Can you work these out from the model? Positions are in its coordinate system, mm. Face numbers are marked on the shaded views. A direction names the side the tool comes from. Give positions to 0.01 mm unless a question says otherwise; leave off trailing zeros. Loops run counter-clockwise (first coordinate to the right, second up) from the corner with the lowest first, then second, coordinate; pieces in that order, holes last. Notation, with made-up numbers: M 18,-20 L 30,-20 A29 ccw 30,17 Z; hole C 85.5,48 d10. An arc over 180 degrees is marked long. Put each result on its own line as item: value. Start each with the question number.
1) Imagine slicing it at D-D (y = -11). Write out the boundary of the cut face in (x, z) (3 decimals), then the cut area to 3 significant figures.
2) Imagine slicing it at B-B (x = 4). Write out the boundary of the cut face in (y, z), then the cut area to 3 significant figures.
3) If we mould it in two halves opening along Y, with no side actions, what happens to the marked faces 4, 5, 6 and 7? For each: +Y half, -Y half, draft (parallel to the pull), parting line (faces both ways), or undercut.
4) Imagine slicing it at C-C (z = 7.75). Write out the boundary of the cut face in (x, y) (3 decimals), then the cut area to 3 significant figures.
5) For the marked faces 1, 2 and 3, which set-ups out of +Z, -Z, +X, -X, +Y, -Y let a thin tool reach every point of the face, with its end or its side?
6) Imagine slicing it at A-A (y = 0). Write out the boundary of the cut face in (x, z) (1 decimal), then the cut area to 3 significant figures.
7) Please list where these lines run through material, in increasing order: line 1 along Z through (x, y) = (32.3, 0); line 2 along X through (y, z) = (-11, 20.75) (3 decimals); line 3 along Z through (x, y) = (17.5, 11). Write a range as from..to.
8) For P1, Ø6, axis at x = 3.5, z = 15, coming from the -Y side; P2, Ø6, axis at y = -31.5, z = 15.5, coming from the +X side; P3, Ø12, axis at x = 12.5, y = 16.5, coming from the -Z side, each with a flat end and sliding along its axis, tell me the tip position at first contact or that it passes through.
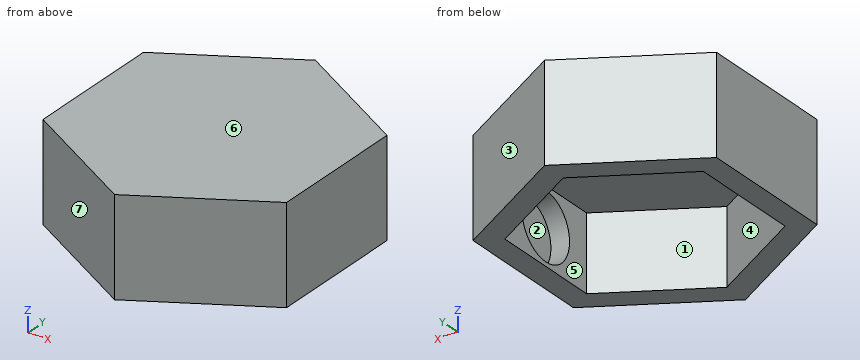
from build123d import *

# Parameters (mm, degrees)
F1_DEPTH = 27.94
F2_T     = -6.477
F3_R     = 9.525
F4_DEPTH = 5.334


with BuildPart() as f1:
    # F0 (on Top) → F1 (new body)
    with BuildSketch(Plane.XY):
        Polygon((34.925, 20.163958), (0, 40.327916), (-34.925, 20.163958), (-34.925, -20.163958), (0, -40.327916), (34.925, -20.163958), align=None)
    extrude(amount=F1_DEPTH)

    # F2
    f2_openings = [f1.faces().sort_by_distance(p)[0] for p in [
        (0, 0, 0),
    ]]
    offset(amount=F2_T, openings=f2_openings)

    # F3 (on face) → F4 (cut)
    with BuildSketch(Plane(origin=(28.448, 0, 0), x_dir=(0, -1, 0), z_dir=(-1, 0, 0))):
        with Locations((0, 10.7315)):
            Circle(F3_R)
    extrude(amount=-F4_DEPTH, mode=Mode.SUBTRACT)


solid = f1.part
Recorded:
1. outline: M -34.925,0 L -28.448,0 L -28.448,21.463 L 28.448,21.463 L 28.448,0 L 34.925,0 L 34.925,27.94 L -34.925,27.94 Z
1. area: 730 mm²
2. outline: M -38.02,0 L -30.54,0 L -30.54,21.46 L 30.54,21.46 L 30.54,0 L 38.02,0 L 38.02,27.94 L -38.02,27.94 Z
2. area: 814 mm²
3. face 4: undercut
3. face 5: undercut
3. face 6: draft
3. face 7: -Y half
4. outline: M -34.925,-20.164 L 0,-40.328 L 34.925,-20.164 L 34.925,20.164 L 0,40.328 L -34.925,20.164 Z; hole M -28.448,-16.424 L 0,-32.849 L 28.448,-16.424 L 28.448,-9.046 L 33.782,-9.046 L 33.782,9.046 L 28.448,9.046 L 28.448,16.424 L 0,32.849 L -28.448,16.424 Z
4. area: 1,330 mm²
5. face 1: -Z
5. face 2: none
5. face 3: +Z, -Z, +X, +Y
6. outline: M -34.9,0 L -28.4,0 L -28.4,21.5 L 28.4,21.5 L 28.4,20.3 L 33.8,20.3 L 33.8,1.2 L 28.4,1.2 L 28.4,0 L 34.9,0 L 34.9,27.9 L -34.9,27.9 Z
6. area: 629 mm²
7. line 1: 0..1.21, 20.26..27.94
7. line 2: -34.925..-28.448, 28.448..34.925
7. line 3: 21.46..27.94
8. P1: y = -40.04
8. P2: x = 20.49
8. P3: z = 21.46
